```python
from build123d import *

# Parameters (mm, degrees)
F0_R      = 10.500004
F1_DEPTH  = 3.499993
F2_R      = 9.45496
F3_DEPTH  = 25.4
F4_R      = 9.45496
F5_DEPTH  = 3.175
F6_R      = 6.000001
F7_DEPTH  = 3.499993
F8_T      = -1.9558
F9_R      = 4.500004
F10_DEPTH = 2514.6


with BuildPart() as f1:
    # F0 (on Top) → F1 (new body)
    with BuildSketch(Plane.XY):
        Circle(F0_R)
    extrude(amount=F1_DEPTH)

    # F2 (on face) → F3 (cut)
    with BuildSketch(Plane.XY.offset(3.499993)):
        Circle(F2_R)
    extrude(amount=-F3_DEPTH, mode=Mode.SUBTRACT)

    # F4 (on Top) → F5 (join)
    with BuildSketch(Plane.XY):
        Circle(F4_R)
    extrude(amount=F5_DEPTH)

    # F6 (on Top) → F7 (join)
    with BuildSketch(Plane.XY):
        Circle(F6_R)
    extrude(amount=F7_DEPTH)

    # F8
    f8_openings = [f1.faces().sort_by_distance(p)[0] for p in [
        (0, 0, 3.499993),
    ]]
    offset(amount=F8_T, openings=f8_openings)

    # F9 (on Top) → F10 (cut)
    with BuildSketch(Plane.XY):
        Circle(F9_R)
    extrude(amount=F10_DEPTH, mode=Mode.SUBTRACT)

    # F11: F1 across plane


with BuildPart() as f1_1:
    add(f1.part)
    add(f1.part.mirror(Plane.XY))


solid = f1_1.part
```
Source: CAD feature listing. Evaluate the final solid. Frame: model axes, mm. A direction names the side the tool comes from. Give positions to 0.01 mm unless a question says otherwise; leave off trailing zeros. Order: outer loops, then holes, each group sorted by start corner. A loop starts at its lowest first (then second) coordinate and runs counter-clockwise, first axis right, second up.
(1) Section query C-C (z = 2). Return the cut outline in (x, y), plus the area to 3 significant figures.
(2) Access query for faces 4 (the face through (-1.4, 4.5, 3.5)), 5 (the face through (5.083, 7.972, 3.34)), 6 (the face through (5.083, 7.972, -3.34)). Directions: +Z, -Z, +X, -X, +Y, -Y. A direction counts if a zero-diameter tool reaches every point of the face in a straight line with its end or side. Return the directions, or none.
(3) Section query D-D (x = 8). Return the cut outline in (y, z) (3 decimals), plus the area to 3 significant figures.
(4) Pull-direction query (Y, two-part tool) for faces 1 (the face through (-2.28, -10.25, 0.05)), 2 (the face through (-9, 4, -3.5)), 3 (the face through (-0.1, -6.2, 3.175)); classes: +Y half, -Y half, draft (parallel to the pull), parting line (faces both ways), or undercut.
(5) Material intervals for line 1 along Y through (x, z) = (0, 3.35); line 2 along Y through (x, z) = (0, 1.75); line 3 along Z through (x, y) = (2.5, 9) (3 decimals), sorted ascending.
(6) Contact query for a flat-ended pin moving along its axis: P1, Ø1, axis at y = -3.5, z = -1.5, coming from the +X side. Output: stop coordinate, or through.
(7) Section query A-A (x = 0). Return the cut outline in (y, z) (3 decimals).
Outcome:
1. outline: circle Ø21 at (0, 0); hole circle Ø9 at (0, 0)
1. area: 283 mm2
2. face 4: +Z, +X, -X, +Y, -Y
2. face 5: +Z
2. face 6: -Z
3. outline: (-6.801, -3.5) - (-5.039, -3.5) - (-5.039, -3.175) - (5.039, -3.175) - (5.039, -3.5) - (6.801, -3.5) - (6.801, 3.5) - (5.039, 3.5) - (5.039, 3.175) - (-5.039, 3.175) - (-5.039, 3.5) - (-6.801, 3.5) - close
3. area: 88.7 mm2
4. face 1: parting line
4. face 2: draft
4. face 3: undercut
5. line 1: y = -10.5 to -9.45, -6 to -4.5, 4.5 to 6, 9.45 to 10.5
5. line 2: y = -10.5 to -4.5, 4.5 to 10.5
5. line 3: z = -3.175 to 3.175
6. P1: stops at x = 10.06
7. outline: (-10.5, -3.5) - (-9.455, -3.5) - (-9.455, -3.175) - (-6, -3.175) - (-6, -3.5) - (-4.5, -3.5) - (-4.5, 3.5) - (-6, 3.5) - (-6, 3.175) - (-9.455, 3.175) - (-9.455, 3.5) - (-10.5, 3.5) - close; (4.5, -3.5) - (6, -3.5) - (6, -3.175) - (9.455, -3.175) - (9.455, -3.5) - (10.5, -3.5) - (10.5, 3.5) - (9.455, 3.5) - (9.455, 3.175) - (6, 3.175) - (6, 3.5) - (4.5, 3.5) - close
